Could you check a few things on this drawing? It's one solid part, dimensions in mm from its lowest x, y, z. A direction names the side the tool comes from. Give positions to 0.01 mm unless a question says otherwise; leave off trailing zeros. Order: outer loops, then holes, each group sorted by start corner. A loop starts at its lowest first (then second) coordinate and runs counter-clockwise, first axis right, second up. Notation, with made-up numbers: (-2.5, 57.5) - (42.5, 57.5) arc R32 ccw to (42.5, 84.5) - close; hole circle Ø11 at (89.25, -7). An arc over 180 degrees is marked (long way). Return JSON: item names as keys, results as strings.
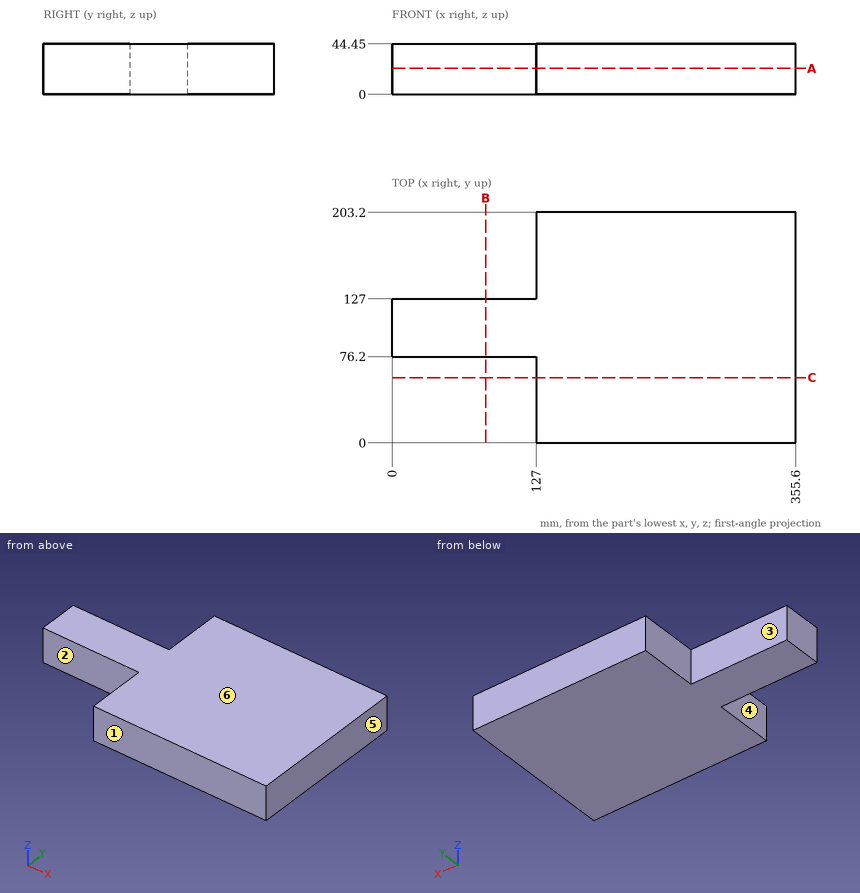
1. If I drill on L1, parallel to X at y = 46.5, z = 2; L2, parallel to Y at x = 53, z = 40.5, over which ranges is the centre line in solid material (lowest first)? Write a range as [from, to].
Checks:
{"L1": "[127, 355.6]", "L2": "[76.2, 127]"}
2. For pin 1 Ø12 at (x, y) = (53.5, 129) entering from +Z; pin 2 Ø13.5 at (x, z) = (94.5, 21) entering from -Y; pin 3 Ø22 at (x, z) = (88.5, 11.5) entering from +Y; pin 4 Ø13.5 at (y, z) = (148.5, 30) entering from -X, each with a flat end and sliding along its axis, tell me the tip position at first contact or that it passes through.
Checks:
{"pin 1": "z = 44.45", "pin 2": "y = 76.2", "pin 3": "y = 127", "pin 4": "x = 127"}
3. Suppose I cut it at C-C (y = 57.5). List the corners of the cut face in (x, z) for me.
Checks:
{"outline": "(127, 0) - (355.6, 0) - (355.6, 44.45) - (127, 44.45) - close"}
4. Thinking about a two-plate mould opening in X: for the marked faces 4, 5 and 6, which applies, +X half, -X half, draft (parallel to the pull), parting line (faces both ways), or undercut?
Checks:
{"face 4": "-X half", "face 5": "+X half", "face 6": "draft"}
5. Suppose I cut it at B-B (x = 82.5). List the corners of the cut face in (y, z) for me.
Checks:
{"outline": "(76.2, 0) - (127, 0) - (127, 44.45) - (76.2, 44.45) - close"}
6. On a 3-axis mill with a long thin cutter (end or side, diameter ignored), from which of +Z, -Z, +X, -X, +Y, -Y can I reach the whole of each face in a straight line? I mean the marked faces 1, 2 and 3. Say none if no direction works.
Checks:
{"face 1": "+Z, -Z, +X, -X, -Y", "face 2": "+Z, -Z, -X, -Y", "face 3": "+Z, -Z, -X, +Y"}
7. Suppose I cut it at A-A (z = 23). List the corners of the cut face in (x, y) for me, plus the area to 3 significant figures.
Checks:
{"outline": "(0, 76.2) - (127, 76.2) - (127, 0) - (355.6, 0) - (355.6, 203.2) - (127, 203.2) - (127, 127) - (0, 127) - close", "area": "52,900 mm^2"}
